The listing builds one solid part. Answer for the finished solid, in the listing's coordinates (mm). Give positions to 0.01 mm unless a question says otherwise; leave off trailing zeros. Loops run counter-clockwise (first coordinate to the right, second up) from the corner with the lowest first, then second, coordinate; pieces in that order, holes last. Notation, with made-up numbers: M 66.25,22 L 92.25,22 A18 ccw 92.25,52 Z; hole C 51,-18 d5. An arc over 180 degrees is marked long. Use one line per item in the form item = value. Start each with the question number.
1. Straight lines are drawn through the part: line 1 (X direction, y = 68.5, z = 2.45); line 2 (Y direction, x = -34.5, z = 1.85); line 3 (X direction, y = 2, z = 3.65). For each, find the intervals that lie inside material, in ascending order. Write a range as from..to.
2. The part is cut by section B-B (x = -15). Write down the section's boundary in (y, z).
3. The part is cut by section D-D (x = -67). Write down the section's boundary in (y, z).
4. The part is cut by section A-A (y = 40). Give the number of separate pieces and of enclosed holes in the cut face, and give its area (3 significant figures).
from build123d import *

# Parameters (mm, degrees)
SALIENTE_EXTRUIR1_DEPTH = 5


with BuildPart() as part:
    # Croquis1 → Saliente-Extruir1 (new body)
    with BuildSketch(Plane.XY):
        Polygon((4.84193268, 80.299895435), (-80.15806732, 80.299895435), (-80.15806732, 42.297370118), (-80.15806732, 28.302420752), (-80.15806732, 21.084166683), (-80.15806732, 7.089217316), (-80.15806732, -9.700104565), (-63.368745439, -9.700104565), (-54.373796072, -9.700104565), (-42.155542003, -9.700104565), (-33.160592637, -9.700104565), (-20.942338567, -9.700104565), (-11.947389201, -9.700104565), (4.84193268, -9.700104565), (4.84193268, 7.089217316), (4.84193268, 21.084166683), (4.84193268, 28.302420752), (4.84193268, 42.297370118), align=None)
        Polygon((-69.477872473, 10.551158094), (-62.406804661, 3.480090282), (-69.477872473, -3.59097753), (-75.15806732, 2.089217316), (-75.15806732, 4.870963247), align=None, mode=Mode.SUBTRACT)
        Polygon((-58.871270756, -0.055443624), (-54.226609815, -4.700104565), (-63.515931696, -4.700104565), align=None, mode=Mode.SUBTRACT)
        Polygon((-75.15806732, 16.23135294), (-73.013406379, 14.086692), (-75.15806732, 11.942031059), align=None, mode=Mode.SUBTRACT)
        Polygon((-58.871270756, 21.157759811), (-51.800202944, 14.086692), (-58.871270756, 7.015624188), (-65.942338567, 14.086692), align=None, mode=Mode.SUBTRACT)
        Polygon((-48.264669038, 10.551158094), (-41.193601226, 3.480090282), (-48.264669038, -3.59097753), (-55.33573685, 3.480090282), align=None, mode=Mode.SUBTRACT)
        Polygon((-37.65806732, -0.055443624), (-33.013406379, -4.700104565), (-42.302728261, -4.700104565), align=None, mode=Mode.SUBTRACT)
        Polygon((-37.65806732, 21.157759811), (-30.586999508, 14.086692), (-37.65806732, 7.015624188), (-44.729135132, 14.086692), align=None, mode=Mode.SUBTRACT)
        Polygon((-69.477872473, 31.764361529), (-62.406804661, 24.693293717), (-69.477872473, 17.622225905), (-75.15806732, 23.302420752), (-75.15806732, 26.084166683), align=None, mode=Mode.SUBTRACT)
        Polygon((-58.871270756, 28.228827623), (-65.942338567, 35.299895435), (-58.871270756, 42.370963247), (-51.800202944, 35.299895435), align=None, mode=Mode.SUBTRACT)
        Polygon((-48.264669038, 31.764361529), (-41.193601226, 24.693293717), (-48.264669038, 17.622225905), (-55.33573685, 24.693293717), align=None, mode=Mode.SUBTRACT)
        Polygon((-27.051465602, 10.551158094), (-19.98039779, 3.480090282), (-27.051465602, -3.59097753), (-34.122533414, 3.480090282), align=None, mode=Mode.SUBTRACT)
        Polygon((-16.444863884, -0.055443624), (-11.800202944, -4.700104565), (-21.089524825, -4.700104565), align=None, mode=Mode.SUBTRACT)
        Polygon((-5.838262167, 10.551158094), (-0.15806732, 4.870963247), (-0.15806732, 2.089217316), (-5.838262167, -3.59097753), (-12.909329978, 3.480090282), align=None, mode=Mode.SUBTRACT)
        Polygon((-16.444863884, 21.157759811), (-9.373796072, 14.086692), (-16.444863884, 7.015624188), (-23.515931696, 14.086692), align=None, mode=Mode.SUBTRACT)
        Polygon((-2.302728261, 14.086692), (-0.15806732, 16.23135294), (-0.15806732, 11.942031059), align=None, mode=Mode.SUBTRACT)
        Polygon((-27.051465602, 31.764361529), (-19.98039779, 24.693293717), (-27.051465602, 17.622225905), (-34.122533414, 24.693293717), align=None, mode=Mode.SUBTRACT)
        Polygon((-5.838262167, 31.764361529), (-0.15806732, 26.084166683), (-0.15806732, 23.302420752), (-5.838262167, 17.622225905), (-12.909329978, 24.693293717), align=None, mode=Mode.SUBTRACT)
        Polygon((-73.013406379, 35.299895435), (-75.15806732, 33.155234494), (-75.15806732, 37.444556376), align=None, mode=Mode.SUBTRACT)
        Polygon((-62.406804661, 45.906497153), (-69.477872473, 38.835429341), (-75.15806732, 44.515624188), (-75.15806732, 47.297370118), (-69.477872473, 52.977564965), align=None, mode=Mode.SUBTRACT)
        Polygon((-44.729135132, 35.299895435), (-37.65806732, 42.370963247), (-30.586999508, 35.299895435), (-37.65806732, 28.228827623), align=None, mode=Mode.SUBTRACT)
        Polygon((-55.33573685, 45.906497153), (-48.264669038, 52.977564965), (-41.193601226, 45.906497153), (-48.264669038, 38.835429341), align=None, mode=Mode.SUBTRACT)
        Polygon((-75.15806732, 58.657759811), (-73.013406379, 56.513098871), (-75.15806732, 54.36843793), align=None, mode=Mode.SUBTRACT)
        Polygon((-65.942338567, 56.513098871), (-58.871270756, 63.584166683), (-51.800202944, 56.513098871), (-58.871270756, 49.442031059), align=None, mode=Mode.SUBTRACT)
        Polygon((-62.406804661, 67.119700589), (-69.477872473, 60.048632777), (-75.15806732, 65.728827623), (-75.15806732, 68.510573554), (-69.477872473, 74.1907684), align=None, mode=Mode.SUBTRACT)
        Polygon((-54.226609815, 75.299895435), (-58.871270756, 70.655234494), (-63.515931696, 75.299895435), align=None, mode=Mode.SUBTRACT)
        Polygon((-44.729135132, 56.513098871), (-37.65806732, 63.584166683), (-30.586999508, 56.513098871), (-37.65806732, 49.442031059), align=None, mode=Mode.SUBTRACT)
        Polygon((-55.33573685, 67.119700589), (-48.264669038, 74.1907684), (-41.193601226, 67.119700589), (-48.264669038, 60.048632777), align=None, mode=Mode.SUBTRACT)
        Polygon((-33.013406379, 75.299895435), (-37.65806732, 70.655234494), (-42.302728261, 75.299895435), align=None, mode=Mode.SUBTRACT)
        Polygon((-34.122533414, 45.906497153), (-27.051465602, 52.977564965), (-19.98039779, 45.906497153), (-27.051465602, 38.835429341), align=None, mode=Mode.SUBTRACT)
        Polygon((-16.444863884, 28.228827623), (-23.515931696, 35.299895435), (-16.444863884, 42.370963247), (-9.373796072, 35.299895435), align=None, mode=Mode.SUBTRACT)
        Polygon((-0.15806732, 33.155234494), (-2.302728261, 35.299895435), (-0.15806732, 37.444556376), align=None, mode=Mode.SUBTRACT)
        Polygon((-0.15806732, 44.515624188), (-5.838262167, 38.835429341), (-12.909329978, 45.906497153), (-5.838262167, 52.977564965), (-0.15806732, 47.297370118), align=None, mode=Mode.SUBTRACT)
        Polygon((-34.122533414, 67.119700589), (-27.051465602, 74.1907684), (-19.98039779, 67.119700589), (-27.051465602, 60.048632777), align=None, mode=Mode.SUBTRACT)
        Polygon((-23.515931696, 56.513098871), (-16.444863884, 63.584166683), (-9.373796072, 56.513098871), (-16.444863884, 49.442031059), align=None, mode=Mode.SUBTRACT)
        Polygon((-0.15806732, 54.36843793), (-2.302728261, 56.513098871), (-0.15806732, 58.657759811), align=None, mode=Mode.SUBTRACT)
        Polygon((-11.800202944, 75.299895435), (-16.444863884, 70.655234494), (-21.089524825, 75.299895435), align=None, mode=Mode.SUBTRACT)
        Polygon((-0.15806732, 68.510573554), (-0.15806732, 65.728827623), (-5.838262167, 60.048632777), (-12.909329978, 67.119700589), (-5.838262167, 74.1907684), align=None, mode=Mode.SUBTRACT)
    extrude(amount=SALIENTE_EXTRUIR1_DEPTH)


solid = part.part
Derived:
q1.line_1 = -80.16..-75.16, -63.79..-53.96, -42.57..-32.74, -21.36..-11.53, -0.16..4.84
q1.line_2 = -9.7..-4.7, -3.21..10.17, 18..31.39, 39.21..52.6, 60.43..73.81, 75.3..80.3
q1.line_3 = -80.16..-75.07, -63.89..-53.86, -42.67..-32.64, -21.46..-11.43, -0.25..4.84
q2.outline = M -9.7,0 L -4.7,0 L -4.7,5 L -9.7,5 Z; M -1.5,0 L 8.46,0 L 8.46,5 L -1.5,5 Z; M 19.71,0 L 29.67,0 L 29.67,5 L 19.71,5 Z; M 40.93,0 L 50.89,0 L 50.89,5 L 40.93,5 Z; M 62.14,0 L 72.1,0 L 72.1,5 L 62.14,5 Z; M 75.3,0 L 80.3,0 L 80.3,5 L 75.3,5 Z
q3.outline = M -9.7,0 L -1.11,0 L -1.11,5 L -9.7,5 Z; M 8.07,0 L 20.1,0 L 20.1,5 L 8.07,5 Z; M 29.29,0 L 41.31,0 L 41.31,5 L 29.29,5 Z; M 50.5,0 L 62.53,0 L 62.53,5 L 50.5,5 Z; M 71.71,0 L 80.3,0 L 80.3,5 L 71.71,5 Z
q4.separate_pieces = 8
q4.enclosed_holes = 0
q4.area = 307 mm2
